from build123d import *

# Parameters (mm, degrees)
SKETCH_1_R      = 7
SKETCH_1_R_2    = 2
SKETCH_1_R_3    = 4.5
SKETCH_1_R_4    = 1.25
EXTRUDE_1_DEPTH = 5


with BuildPart() as part:
    # 草图1 → 凸台-拉伸1 (new body)
    with BuildSketch(Plane(origin=(0, 0, 0), x_dir=(1, 0, 0), z_dir=(0, 1, 0))):
        with BuildLine():
            Line((-65.328738569, 31.45065883), (-65.328738569, -58.54934117))
            Line((-65.328738569, -58.54934117), (-55.328738569, -58.54934117))
            Line((-55.328738569, -58.54934117), (-15.328738569, -58.54934117))
            Line((-15.328738569, -58.54934117), (-5.328738569, -58.54934117))
            Line((-5.328738569, -58.54934117), (-5.328738569, 2.36065883))
            Line((-5.328738569, 2.36065883), (-5.328738569, 31.45065883))
            ThreePointArc((-5.328738569, 31.45065883), (-8.257670757, 38.521726641), (-15.328738569, 41.45065883))
            Line((-15.328738569, 41.45065883), (-55.328738569, 41.45065883))
            ThreePointArc((-55.328738569, 41.45065883), (-62.399806381, 38.521726641), (-65.328738569, 31.45065883))
        make_face()
        with Locations(Location((-49.728738569, 2.36065883, 0), (0, 0, 270))):
            Circle(SKETCH_1_R, mode=Mode.SUBTRACT)
        with Locations(Location((-55.328738569, -53.54934117, 0), (0, 0, 270))):
            Circle(SKETCH_1_R_2, mode=Mode.SUBTRACT)
        with Locations(Location((-15.328738569, -53.54934117, 0), (0, 0, 270))):
            Circle(SKETCH_1_R_2, mode=Mode.SUBTRACT)
        with Locations(Location((-15.328738569, 26.45065883, 0), (0, 0, 270))):
            Circle(SKETCH_1_R_3, mode=Mode.SUBTRACT)
        with Locations(Location((-54.228738569, 17.36065883, 0), (0, 0, 270))):
            Circle(SKETCH_1_R_4, mode=Mode.SUBTRACT)
        with Locations(Location((-37.228738569, 17.36065883, 0), (0, 0, 270))):
            Circle(SKETCH_1_R_4, mode=Mode.SUBTRACT)
        with Locations(Location((-20.228738569, 17.36065883, 0), (0, 0, 270))):
            Circle(SKETCH_1_R_4, mode=Mode.SUBTRACT)
        with Locations(Location((-54.228738569, -12.63934117, 0), (0, 0, 270))):
            Circle(SKETCH_1_R_4, mode=Mode.SUBTRACT)
        with Locations(Location((-37.228738569, -12.63934117, 0), (0, 0, 270))):
            Circle(SKETCH_1_R_4, mode=Mode.SUBTRACT)
        with Locations(Location((-20.228738569, -12.63934117, 0), (0, 0, 270))):
            Circle(SKETCH_1_R_4, mode=Mode.SUBTRACT)
    extrude(amount=EXTRUDE_1_DEPTH)


solid = part.part
Geometry: final body of the model. Coordinates: model frame, mm. Round coordinates to 2 decimals unless told otherwise and drop trailing zeros. Loops run counter-clockwise (first coordinate to the right, second up) from the corner with the lowest first, then second, coordinate; pieces in that order, holes last. Notation, with made-up numbers: (11, 30) -> (59, 30) arc R19 cw to (59, 38) -> close; hole circle Ø6 at (-39.75, 53.25). An arc over 180 degrees is marked (long way). One line per question, with ' | ' between items. Start each with the question number.
1. Section C-C on z = -1. Output: boundary loops of the cut face in (x, y).
2. Section B-B on y = 1.5. Count the separate pieces of the cut face and the enclosed holes in it, and give its area (3 significant figures).
3. Line query: line 1 along Z through (x, y) = (-12.5, 3.05); line 2 along Z through (x, y) = (-47.5, 1.3); line 3 along X through (y, z) = (4.85, -23). Output: solid intervals per line, ascending. Write a range as [from, to].
4. Mould query, pull axis X, two halves, no side actions, for faces 1 (the face through (-36, 5, 8)), 2 (the face through (-62.32, 2.46, -38.6)), 3 (the face through (-55.45, 2.46, 12.37)). Classes: pulls with the +X half, pulls with the -X half, needs draft (parallel to the pull), parting line crosses it, or undercut.
5. Section A-A on x = -48.5. Output: boundary loops of the cut face in (y, z).
Returned:
1) outline: (-65.33, 0) -> (-56.6, 0) -> (-56.6, 5) -> (-65.33, 5) -> close; (-42.86, 0) -> (-5.33, 0) -> (-5.33, 5) -> (-42.86, 5) -> close
2) separate pieces: 1 | enclosed holes: 10 | area: 5,680 mm2
3) line 1: z = [-41.04, -29.95], [-22.95, 58.55] | line 2: z = [-41.45, -9], [4.28, 58.55] | line 3: x = [-65.33, -18.22], [-12.44, -5.33]
4) face 1: needs draft | face 2: pulls with the -X half | face 3: undercut
5) outline: (0, -41.45) -> (5, -41.45) -> (5, -9.25) -> (0, -9.25) -> close; (0, 4.53) -> (5, 4.53) -> (5, 58.55) -> (0, 58.55) -> close
